from build123d import *

# Parameters (mm, degrees)
F1_DEPTH = 1.016
F2_SIZE  = 1.01599


# Not quite as in the source:
# - a fillet or chamfer is up to 0.001 mm smaller than in the source, because OpenCascade refuses the exact size


with BuildPart() as f1:
    # F0 (on Top) → F1 (new body)
    with BuildSketch(Plane.XY):
        with BuildLine():
            ThreePointArc((0, 2.9195159057), (0.527538065, 2.8714589869), (1.0377089673, 2.7288703199))
            Line((1.0377089673, 2.7288703199), (1.0377089673, 31.7330373601))
            Line((1.0377089673, 31.7330373601), (-1.4246536514, 31.7180210917))
            Line((-1.4246536514, 31.7180210917), (-1.4426441077, 7.0411415527))
            Line((-1.4426441077, 7.0411415527), (0, 5.0220009871))
            Line((0, 5.0220009871), (0, 2.9195159057))
        make_face()
        with BuildLine():
            Line((1.0377089673, 1.7452047762), (1.0377089673, 2.7288703199))
            ThreePointArc((1.0377089673, 2.7288703199), (0.527538065, 2.8714589869), (0, 2.9195159057))
            Line((0, 2.9195159057), (1.0377089673, 1.7452047762))
        make_face()
        with BuildLine():
            Line((1.7452047762, -1.0377089673), (2.9195159057, 0))
            ThreePointArc((2.9195159057, 0), (2.4034538646, 1.6574023784), (1.0377089673, 2.7288703199))
            Line((1.0377089673, 2.7288703199), (1.0377089673, 1.7452047762))
            Line((1.0377089673, 1.7452047762), (0, 2.9195159057))
            ThreePointArc((0, 2.9195159057), (-1.6574023784, 2.4034538646), (-2.7288703199, 1.0377089673))
            Line((-2.7288703199, 1.0377089673), (-1.7452047762, 1.0377089673))
            Line((-1.7452047762, 1.0377089673), (-2.9195159057, 0))
            ThreePointArc((-2.9195159057, 0), (-2.4034538646, -1.6574023784), (-1.0377089673, -2.7288703199))
            Line((-1.0377089673, -2.7288703199), (-1.0377089673, -1.7452047762))
            Line((-1.0377089673, -1.7452047762), (0, -2.9195159057))
            ThreePointArc((0, -2.9195159057), (1.6574023784, -2.4034538646), (2.7288703199, -1.0377089673))
            Line((2.7288703199, -1.0377089673), (1.7452047762, -1.0377089673))
        make_face()
        with BuildLine():
            Line((-1.7452047762, 1.0377089673), (-2.7288703199, 1.0377089673))
            ThreePointArc((-2.7288703199, 1.0377089673), (-2.8714589869, 0.527538065), (-2.9195159057, 0))
            Line((-2.9195159057, 0), (-1.7452047762, 1.0377089673))
        make_face()
        with BuildLine():
            ThreePointArc((2.7288703199, -1.0377089673), (2.8714589869, -0.527538065), (2.9195159057, 0))
            Line((2.9195159057, 0), (1.7452047762, -1.0377089673))
            Line((1.7452047762, -1.0377089673), (2.7288703199, -1.0377089673))
        make_face()
        with BuildLine():
            Line((5.0220009871, 0), (2.9195159057, 0))
            ThreePointArc((2.9195159057, 0), (2.8714589869, -0.527538065), (2.7288703199, -1.0377089673))
            Line((2.7288703199, -1.0377089673), (31.7330373601, -1.0377089673))
            Line((31.7330373601, -1.0377089673), (31.7180210917, 1.4246536514))
            Line((31.7180210917, 1.4246536514), (7.0411415527, 1.4426441077))
            Line((7.0411415527, 1.4426441077), (5.0220009871, 0))
        make_face()
        with BuildLine():
            ThreePointArc((-1.0377089673, -2.7288703199), (-0.527538065, -2.8714589869), (0, -2.9195159057))
            Line((0, -2.9195159057), (-1.0377089673, -1.7452047762))
            Line((-1.0377089673, -1.7452047762), (-1.0377089673, -2.7288703199))
        make_face()
        with BuildLine():
            Line((0, -5.0220009871), (0, -2.9195159057))
            ThreePointArc((0, -2.9195159057), (-0.527538065, -2.8714589869), (-1.0377089673, -2.7288703199))
            Line((-1.0377089673, -2.7288703199), (-1.0377089673, -31.7330373601))
            Line((-1.0377089673, -31.7330373601), (1.4246536514, -31.7180210917))
            Line((1.4246536514, -31.7180210917), (1.4426441077, -7.0411415527))
            Line((1.4426441077, -7.0411415527), (0, -5.0220009871))
        make_face()
        with BuildLine():
            ThreePointArc((-2.9195159057, 0), (-2.8714589869, 0.527538065), (-2.7288703199, 1.0377089673))
            Line((-2.7288703199, 1.0377089673), (-31.7330373601, 1.0377089673))
            Line((-31.7330373601, 1.0377089673), (-31.7180210917, -1.4246536514))
            Line((-31.7180210917, -1.4246536514), (-7.0411415527, -1.4426441077))
            Line((-7.0411415527, -1.4426441077), (-5.0220009871, 0))
            Line((-5.0220009871, 0), (-2.9195159057, 0))
        make_face()
    extrude(amount=F1_DEPTH)

    # F2 (size 1.016 in the source; OpenCascade refuses exactly that, so slightly less here)
    f2_edges = [f1.edges().sort_by_distance(p)[0] for p in [
        (-19.379581, -1.433649, 1.016),
        (1.433649, -19.379581, 1.016),
        (19.379581, 1.433649, 1.016),
        (-1.433649, 19.379581, 1.016),
    ]]
    chamfer(f2_edges, length=F2_SIZE)


solid = f1.part
Design review of the part built by this model. Coordinates are the model's own, in mm. A direction names the side the tool comes from. Coordinates: 2 decimals unless noted, no trailing zeros. Order: outer loops, then holes, each group sorted by start corner. A loop starts at its lowest first (then second) coordinate and runs counter-clockwise, first axis right, second up.
Item 1: For pin 1 Ø0.5 at (x, z) = (4.5, 0.5) entering from +Y; pin 2 Ø0.5 at (x, z) = (-21, 0.5) entering from +Y, all flat-tipped, find the tip position at first contact; note any pin that passes through.
Item 2: The part is to be moulded in two halves that separate along X. For faces 1 (the cylindrical face through (-1.637, 2.417, 0.501)), 2 (the flat face through (0.57, -5.82, 0.39)), 3 (the cylindrical face through (-2.417, -1.637, 0.501)), say which applies: pulls with the +X half, pulls with the -X half, needs draft (parallel to the pull), parting line crosses it, or undercut.
Item 3: Take a section at C-C, the plane z = 0.55. Write out the cut boundary in (x, y), then the cut area to 3 significant figures.
Item 4: For line 1 (Y direction, x = -12, z = 0.4); line 2 (X direction, y = -5, z = 0.9); line 3 (Y direction, x = 1, z = 0.9), list the stretches that pass through material, from the lowest coordinate up.
Item 5: For faces 4 (the flat face through (-0.57, 5.82, 0.39)), 5 (the cylindrical face through (1.637, -2.417, 0.501)), 6 (the flat face through (5.82, 0.57, 0.39)), 7 (the flat face through (-5.82, -0.57, 0.39)), list the 3-axis set-ups (+Z, -Z, +X, -X, +Y, -Y) from which the entire face can be reached by the end or side of a thin tool; tool diameter is ignored.
The answers:
1. pin 1: stops at y = 0
1. pin 2: stops at y = 1.04
2. face 1: pulls with the -X half
2. face 2: pulls with the +X half
2. face 3: undercut
3. outline: (-31.73, 1.04) - (-31.72, -0.87) - (-6.27, -0.89) - (-5.02, 0) - (-2.92, 0) arc R2.92 ccw to (-1.04, -2.73) - (-1.04, -31.73) - (0.87, -31.72) - (0.89, -6.27) - (0, -5.02) - (0, -2.92) arc R2.92 ccw to (2.73, -1.04) - (31.73, -1.04) - (31.72, 0.87) - (6.27, 0.89) - (5.02, 0) - (2.92, 0) arc R2.92 ccw to (1.04, 2.73) - (1.04, 31.73) - (-0.87, 31.72) - (-0.89, 6.27) - (0, 5.02) - (0, 2.92) arc R2.92 ccw to (-2.73, 1.04) - close
3. area: 239 mm2
4. line 1: y = -1.04 to 1.04
4. line 2: x = -1.04 to 0
4. line 3: y = -2.74 to 31.73
5. face 4: +Z, -Z, -X
5. face 5: +Z, -Z, +X
5. face 6: +Z, -Z, +Y
5. face 7: +Z, -Z, -Y
